Geometry: see drawing. Coordinates: mm, zero at the bounding-box minimum. A direction names the side the tool comes from. Coordinates: 2 decimals unless noted, no trailing zeros. Loops run counter-clockwise (first coordinate to the right, second up) from the corner with the lowest first, then second, coordinate; pieces in that order, holes last. Notation, with made-up numbers: (17.5, -21) - (75.5, -21) arc R23 cw to (75.5, -11) - close; hole circle Ø2 at (5.25, 31.25). An arc over 180 degrees is marked (long way). Write each question's results on one line, items separated by ' | '. Start each with the question number.
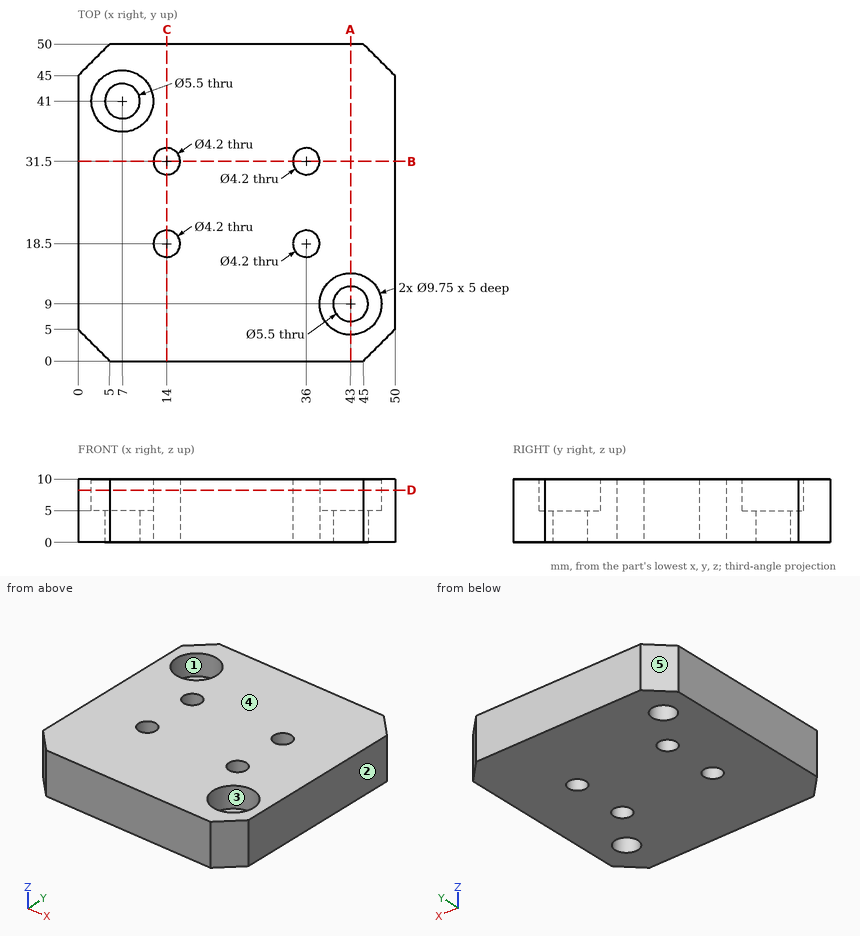
1) Section query A-A on x = 43. Output: boundary loops of the cut face in (y, z) (3 decimals).
2) Pull-direction query (Y, two-part tool) for the marked faces 3, 4 and 5; classes: released by +Y, released by -Y, zero draft, split by the parting line, or undercut.
3) Access query for the marked faces 1 and 2. Directions: +Z, -Z, +X, -X, +Y, -Y. A direction counts if a zero-diameter tool reaches every point of the face in a straight line with its end or side. Return the directions, or none.
4) Section query D-D on z = 8.25. Output: boundary loops of the cut face in (x, y) (3 decimals).
5) Pin query (flat end, axial travel): pin 1 Ø6.5 at (x, y) = (43, 9) entering from +Z. Return the tip coordinate at first contact, or that it passes through.
6) Section query B-B on y = 31.5. Output: boundary loops of the cut face in (x, z), and give its area (3 significant figures).
7) Section query C-C on x = 14. Output: boundary loops of the cut face in (y, z).
8) Material intervals for line 1 (X direction, y = 18.5, z = 5.5); line 2 (Y direction, x = 14, z = 7.75); line 3 (X direction, y = 41, z = 7.3) (3 decimals), sorted ascending. Write a range as [from, to].
Returned:
1) outline: (0, 0) - (6.25, 0) - (6.25, 5) - (4.125, 5) - (4.125, 10) - (0, 10) - close; (11.75, 0) - (50, 0) - (50, 10) - (13.875, 10) - (13.875, 5) - (11.75, 5) - close
2) face 3: undercut | face 4: zero draft | face 5: released by +Y
3) face 1: +Z | face 2: +Z, -Z, +X, +Y, -Y
4) outline: (0, 5) - (5, 0) - (45, 0) - (50, 5) - (50, 45) - (45, 50) - (5, 50) - (0, 45) - close; hole circle Ø9.75 at (7, 41); hole circle Ø4.2 at (14, 18.5); hole circle Ø4.2 at (14, 31.5); hole circle Ø4.2 at (36, 18.5); hole circle Ø4.2 at (36, 31.5); hole circle Ø9.75 at (43, 9)
5) pin 1: stops at z = 5
6) outline: (0, 0) - (11.9, 0) - (11.9, 10) - (0, 10) - close; (16.1, 0) - (33.9, 0) - (33.9, 10) - (16.1, 10) - close; (38.1, 0) - (50, 0) - (50, 10) - (38.1, 10) - close | area: 416 mm²
7) outline: (0, 0) - (16.4, 0) - (16.4, 10) - (0, 10) - close; (20.6, 0) - (29.4, 0) - (29.4, 10) - (20.6, 10) - close; (33.6, 0) - (50, 0) - (50, 10) - (33.6, 10) - close
8) line 1: x = [0, 11.9], [16.1, 33.9], [38.1, 50] | line 2: y = [0, 16.4], [20.6, 29.4], [33.6, 50] | line 3: x = [0, 2.125], [11.875, 50]
